Source: CAD feature listing. Evaluate the final solid. Frame: model axes, mm. A direction names the side the tool comes from. Coordinates: 2 decimals unless noted, no trailing zeros. Write each loop counter-clockwise with the first axis right and the second up, starting at its lowest first coordinate (ties: lowest second). Pieces come first, ordered by that corner, then holes. Notation, with made-up numbers: M 30.25,24 L 85.25,24 A17 cw 85.25,45 Z; hole C -25,-6.75 d7. An arc over 180 degrees is marked long. One line per item, written item: value. Start each with the question number.
Item 1: Cut plane B-B, the plane x = -4. Output: boundary loops of the cut face in (y, z), then the cut area to 3 significant figures.
Item 2: Cut plane D-D, the plane y = 11. Output: boundary loops of the cut face in (x, z), then the cut area to 3 significant figures.
Item 3: Cut plane A-A, the plane z = 0. Output: boundary loops of the cut face in (x, y) (3 decimals).
Item 4: Pin query (flat end, axial travel): P1, Ø3, axis at y = 3.5, z = -13.5, coming from the +X side; P2, Ø6.5, axis at x = -1.5, z = 16, coming from the +Y side; P3, Ø10, axis at x = -5.5, z = 14.5, coming from the -Y side; P4, Ø9.5, axis at x = 0, z = 0, coming from the -Y side. Return the tip coordinate at first contact, or that it passes through.
Item 5: Cut plane C-C, the plane x = 0. State how many separate pieces and enclosed holes the cut face has, then the cut area to 3 significant figures.
Item 6: Mould query, pull axis X, two halves, no side actions, for faces 1 (the cylindrical face through (-1.69, -0.62, 7.59)), 2 (the cylindrical face through (-0.38, 3.76, -18.3)), 3 (the flat face through (4, -1.25, -5)), 4 (the cylindrical face through (-12.3, 2.3, 0.2)). Classes: released by +X, released by -X, zero draft, split by the parting line, or undercut.
Item 7: Set-up query: faces 5 (the flat face through (-8, 0, 0)), 6 (the flat face through (4.5, 2, -13)), 7 (the flat face through (-4.5, 2, 13)), 8 (the flat face through (5, 4.75, -10)). Return all of +Z, -Z, +X, -X, +Y, -Y with unobstructed straight access to the full face (end or side cutting, diameter ignored); none if empty.
Item 8: Ray query, L1, parallel to Z at x = 0, y = 1.7 (3 decimals); L2, parallel to Z at x = 0, y = 4.05 (3 decimals); L3, parallel to Z at x = 0, y = 9. Return the intervals inside material, ascending. Write a range as from..to.
Autodesk Inventor part; units mm, degrees
ref_plane "YZ Plane" through (0, 0, 0) normal (1, 0, 0) x (0, 1, 0)
ref_plane "XZ Plane" through (0, 0, 0) normal (0, 1, 0) x (-1, 0, 0)
ref_plane "XY Plane" through (0, 0, 0) normal (0, 0, 1) x (1, 0, 0)
sketch "Esboço1" plane through (0, 0, 0) normal (0, 1, 0) x (-1, 0, 0)
  circle A0 centre (0, 0) radius 12.3
  dimension "d0" = 24.6
extrude "Extrusão1" add sketch "Esboço1" along normal blind 4.75
sketch "Esboço2" plane through (0, 0, 0) normal (0, -1, 0) x (1, 0, 0)
  circle A0 centre (0, 0) radius 7.775
  dimension "d3" = 15.55
extrude "Extrusão2" add sketch "Esboço2" along normal blind 1.25
sketch "Esboço3" plane through (0, 0, 0) normal (0, -1, 0) x (1, 0, 0)
  circle A0 centre (0, 0) radius 12.3
  circle A1 centre (0, -15.425) radius 1.25
  line L0 (-4.5, -15.425) -> (-4.5, -11.4473)
  line L1 (4.5, -15.425) -> (4.5, -11.4473)
  line L2 (4.5, -15.425) -> (8.4777, -15.425) construction
  arc A2 (-4.5, -15.425) -> (4.5, -15.425) centre (0, -15.425) ccw
  dimension "d12" = 90
extrude "Extrusão3" add sketch "Esboço3" against normal blind 4.75 contours A0 L1 A2 L0
sketch "Esboço4" plane through (0, 4.75, 0) normal (0, 1, 0) x (1, 0, 0)
  circle A0 centre (0, 15.425) radius 1.25
  circle A1 centre (0, 15.425) radius 2.9
  point P0 (0, 0)
  dimension "d15" = 5.8
extrude "Extrusão4" cut sketch "Esboço4" against normal blind 2
pattern_circular "Padrão circular1" count 2 over 360 about axis through (0, 0, 0) along (0, 1, 0) of "Extrusão3", "Extrusão4"
sketch "Esboço5" plane through (0, 4.75, 0) normal (0, 1, 0) x (1, 0, 0)
  circle A0 centre (0, 0) radius 11
  dimension "d21" = 22
extrude "Extrusão5" add sketch "Esboço5" along normal blind 12
sketch "Esboço6" plane through (0, 16.75, 0) normal (0, 1, 0) x (1, 0, 0)
  circle A0 centre (0, 0) radius 6
  dimension "d24" = 12
extrude "Extrusão6" cut sketch "Esboço6" against normal blind 20
thread "Rosca1"
sketch "Esboço7" plane through (0, 0, 0) normal (0, -1, 0) x (1, 0, 0)
  circle A0 centre (0, -15.425) radius 1.25
  circle A1 centre (0, -15.425) radius 1.5
  circle A2 centre (0, 15.425) radius 1.25
  circle A3 centre (0, 15.425) radius 1.5
  circle A4 centre (0, 0) radius 8
  line L0 (-14, 21.425) -> (14, 21.425)
  line L1 (14, 21.425) -> (14, -21.425)
  line L2 (14, -21.425) -> (-14, -21.425)
  line L3 (-14, -21.425) -> (-14, 21.425)
  dimension "d29" = 3
  dimension "d30" = 3
  dimension "d31" = 16
properties part number "prensa_cabo_fixador"
From the geometry:
1. outline: M -1.25,-6.67 L 0,-6.67 L 0,-17.49 L 4.75,-17.49 L 4.75,-10.25 L 16.75,-10.25 L 16.75,-4.47 L -1.25,-4.47 Z; M -1.25,4.47 L 16.75,4.47 L 16.75,10.25 L 4.75,10.25 L 4.75,17.49 L 0,17.49 L 0,6.67 L -1.25,6.67 Z
1. area: 268 mm²
2. outline: C 0,0 d22; hole C 0,0 d12
2. area: 267 mm²
3. outline: M -12.3,0 L -7.775,0 L -7.775,-1.25 L -6,-1.25 L -6,16.75 L -11,16.75 L -11,4.75 L -12.3,4.75 Z; M 6,-1.25 L 7.775,-1.25 L 7.775,0 L 12.3,0 L 12.3,4.75 L 11,4.75 L 11,16.75 L 6,16.75 Z
4. P1: stops at x = 4.5
4. P2: stops at y = 4.75
4. P3: stops at y = 0
4. P4: passes through
5. separate pieces: 4
5. enclosed holes: 0
5. area: 220 mm²
6. face 1: split by the parting line
6. face 2: undercut
6. face 3: zero draft
6. face 4: released by -X
7. face 5: -Y
7. face 6: -Z, +X, +Y, -Y
7. face 7: +Z, -X, +Y, -Y
7. face 8: +Y
8. L1: z = -19.925..-16.675, -14.175..-6, 6..14.175, 16.675..19.925
8. L2: z = -19.925..-18.325, -12.525..-6, 6..12.525, 18.325..19.925
8. L3: z = -11..-6, 6..11
